Input: part model. Units: mm. Frame: model coordinates. A direction names the side the tool comes from. Round coordinates to 2 decimals unless told otherwise and drop trailing zeros. Loops run counter-clockwise (first coordinate to the right, second up) from the corner with the lowest first, then second, coordinate; pieces in that order, holes last. Notation, with made-up numbers: (51, 81.5) -> (55, 81.5) arc R25 cw to (55, 99.5) -> close; hole circle Ø9 at (38, -8). An arc over 180 degrees is marked (long way). Answer as a JSON object with one key per item and string values. Group by question number.
Item 1: Material intervals for line 1 (X direction, y = 28, z = 0); line 2 (Z direction, x = 49, y = 1.6); line 3 (Y direction, x = 0, z = -33), sorted ascending. Write a range as [from, to].
Item 2: Section query B-B on x = -11. Return loops of the section in (y, z), and give its area (3 significant figures).
Item 3: Pin query (flat end, axial travel): pin 1 (4 mm diameter, centred on y = 13, z = 25, fed in from -X); pin 2 (1.9 mm diameter, centred on x = -49, z = -34.75, fed in from +Y); pin 3 (12 mm diameter, centred on x = 8, z = 0, fed in from -Y). Return the tip coordinate at first contact, or that it passes through.
Item 4: Section query C-C on y = 27. Return loops of the section in (x, z).
Item 5: Draft query along Z for faces 1 (the flat face through (4, 1, 50)), 2 (the flat face through (2, 2, -44)), 3 (the flat face through (3, 2, 0)). Return one class per face: released by +Z, released by -Z, zero draft, split by the parting line, or undercut.
Item 6: Section query A-A on z = 22. Return loops of the section in (x, y), and give its area (3 significant figures).
Item 7: Set-up query: faces 4 (the cylindrical face through (29.061, 15.804, -31.693)), 5 (the flat face through (0, 0, 12)), 6 (the flat face through (-38, 30, 13)). Return all of +Z, -Z, +X, -X, +Y, -Y with unobstructed straight access to the full face (end or side cutting, diameter ignored); none if empty.
from build123d import *

# Parameters (mm, degrees)
CROQUIS1_R              = 43
CROQUIS1_R_2            = 40
SALIENTE_EXTRUIR1_DEPTH = 30
CROQUIS3_R              = 0.81
CROQUIS3_R_2            = 2
SALIENTE_EXTRUIR2_DEPTH = 2
CROQUIS4_W              = 140
CROQUIS4_H              = 100
CROQUIS4_R              = 43
SALIENTE_EXTRUIR3_DEPTH = 2
CROQUIS5_R              = 0.81
CORTAR_EXTRUIR1_DEPTH   = 2
SALIENTE_EXTRUIR7_DEPTH = 25
MATRIZL1_COUNT          = 2
MATRIZL1_PITCH          = 50


with BuildPart() as part:
    # Croquis1 → Saliente-Extruir1 (new body)
    with BuildSketch(Plane(origin=(0, 0, 0), x_dir=(1, 0, 0), z_dir=(0, 1, 0))):
        with Locations(Location((0, 0, 0), (0, 0, 270))):
            Circle(CROQUIS1_R)
        with Locations(Location((0, 0, 0), (0, 0, 270))):
            Circle(CROQUIS1_R_2, mode=Mode.SUBTRACT)
    extrude(amount=SALIENTE_EXTRUIR1_DEPTH)

    # Croquis3 → Saliente-Extruir2 (add)
    with BuildSketch(Plane(origin=(0, 0, 0), x_dir=(1, 0, 0), z_dir=(0, 1, 0))):
        with BuildLine():
            Line((-2, 39.949968711), (-2, 2))
            Line((-2, 2), (-39.949968711, 2))
            ThreePointArc((-39.949968711, 2), (-40, 0), (-39.949968711, -2))
            Line((-39.949968711, -2), (-2, -2))
            Line((-2, -2), (-2, -39.949968711))
            ThreePointArc((-2, -39.949968711), (0, -40), (2, -39.949968711))
            Line((2, -39.949968711), (2, -2))
            Line((2, -2), (39.949968711, -2))
            ThreePointArc((39.949968711, -2), (39.987490222, -1.000312842), (40, 0))
            ThreePointArc((40, 0), (39.987490222, 1.000312842), (39.949968711, 2))
            Line((39.949968711, 2), (2, 2))
            Line((2, 2), (2, 39.949968711))
            ThreePointArc((2, 39.949968711), (0, 40), (-2, 39.949968711))
        make_face()
        with Locations(Location((0, -4.5, 0), (0, 0, 270))):
            Circle(CROQUIS3_R, mode=Mode.SUBTRACT)
        with Locations(Location((-4.5, 0, 0), (0, 0, 270))):
            Circle(CROQUIS3_R, mode=Mode.SUBTRACT)
        with Locations(Location((0, 0, 0), (0, 0, 270))):
            Circle(CROQUIS3_R_2, mode=Mode.SUBTRACT)
        with Locations(Location((4.5, 0, 0), (0, 0, 270))):
            Circle(CROQUIS3_R, mode=Mode.SUBTRACT)
        with Locations(Location((0, 4.5, 0), (0, 0, 270))):
            Circle(CROQUIS3_R, mode=Mode.SUBTRACT)
    extrude(amount=SALIENTE_EXTRUIR2_DEPTH)

    # Croquis4 → Saliente-Extruir3 (add)
    with BuildSketch(Plane(origin=(0, 0, 0), x_dir=(1, 0, 0), z_dir=(0, 1, 0))):
        Rectangle(CROQUIS4_W, CROQUIS4_H)
        with Locations(Location((0, 0, 0), (0, 0, 90))):
            Circle(CROQUIS4_R, mode=Mode.SUBTRACT)
    extrude(amount=SALIENTE_EXTRUIR3_DEPTH)

    # Croquis5 → Cortar-Extruir1 (cut)
    with BuildSketch(Plane(origin=(0, 2, 0), x_dir=(1, 0, 0), z_dir=(0, 1, 0))):
        with Locations(Location((-68, -34.75, 0), (0, 0, 270))):
            Circle(CROQUIS5_R)
        with Locations(Location((-49, -34.75, 0), (0, 0, 270))):
            Circle(CROQUIS5_R)
        with Locations(Location((-49, 34.75, 0), (0, 0, 90))):
            Circle(CROQUIS5_R)
        with Locations(Location((-68, 34.75, 0), (0, 0, 90))):
            Circle(CROQUIS5_R)
        with Locations(Location((68, 34.75, 0), (0, 0, 270))):
            Circle(CROQUIS5_R)
        with Locations(Location((49, 34.75, 0), (0, 0, 270))):
            Circle(CROQUIS5_R)
        with Locations(Location((49, -34.75, 0), (0, 0, 90))):
            Circle(CROQUIS5_R)
        with Locations(Location((68, -34.75, 0), (0, 0, 90))):
            Circle(CROQUIS5_R)
    extrude(amount=-CORTAR_EXTRUIR1_DEPTH, mode=Mode.SUBTRACT)

    # Croquis7 → Saliente-Extruir7 (add)
    with BuildSketch(Plane.XY.offset(50)):
        with BuildLine():
            Line((70, 2), (70, 0))
            Line((70, 0), (71.227232035, 0))
            ThreePointArc((71.227232035, 0), (77.518734657, 4.645751311), (69.872983346, 3))
            Line((69.872983346, 3), (70.872983346, 3))
            ThreePointArc((70.872983346, 3), (76.829779025, 3.507305936), (71.044556221, 2))
            Line((71.044556221, 2), (70, 2))
        make_face()
    saliente_extruir7 = extrude(amount=-SALIENTE_EXTRUIR7_DEPTH)

    # MatrizL1: Saliente-Extruir7 ×2
    with Locations(*[(0, 0, -i * MATRIZL1_PITCH) for i in range(1, MATRIZL1_COUNT)]):
        add(saliente_extruir7)


solid = part.part
Solved:
{
 "1": {"line 1": "[-43, -40], [40, 43]", "line 2": "[-50, -35.56], [-33.94, 33.94], [35.56, 50]", "line 3": "[0, 2]"},
 "2": {"outline": "(0, -50) -> (2, -50) -> (2, -41.57) -> (30, -41.57) -> (30, -38.46) -> (0, -38.46) -> close; (0, -2) -> (2, -2) -> (2, 2) -> (0, 2) -> close; (0, 38.46) -> (30, 38.46) -> (30, 41.57) -> (2, 41.57) -> (2, 50) -> (0, 50) -> close", "area": "228 mm²"},
 "3": {"pin 1": "x = -36.33", "pin 2": "y = 2", "pin 3": "y = 0"},
 "4": {"outline": "circle Ø86 at (0, 0); hole circle Ø80 at (0, 0)"},
 "5": {"face 1": "released by +Z", "face 2": "zero draft", "face 3": "undercut"},
 "6": {"outline": "(-70, 0) -> (-33.41, 0) -> (-33.41, 30) -> (-36.95, 30) -> (-36.95, 2) -> (-70, 2) -> close; (-2, 0) -> (2, 0) -> (2, 2) -> (-2, 2) -> close; (33.41, 0) -> (70, 0) -> (70, 2) -> (36.95, 2) -> (36.95, 30) -> (33.41, 30) -> close", "area": "353 mm²"},
 "7": {"face 4": "+Y", "face 5": "+Z, -Z, -X, -Y", "face 6": "+Z, -Z, +X, -X, +Y"}
}
